Answer from the drawing. Dimensions are ordinates in mm from the lowest x, y and z of the part. A direction names the side the tool comes from. Give positions to 0.01 mm unless a question says otherwise; leave off trailing zeros. Write each loop counter-clockwise with the first axis right and the second up, starting at its lowest first coordinate (ties: lowest second). Pieces come first, ordered by that corner, then holes.
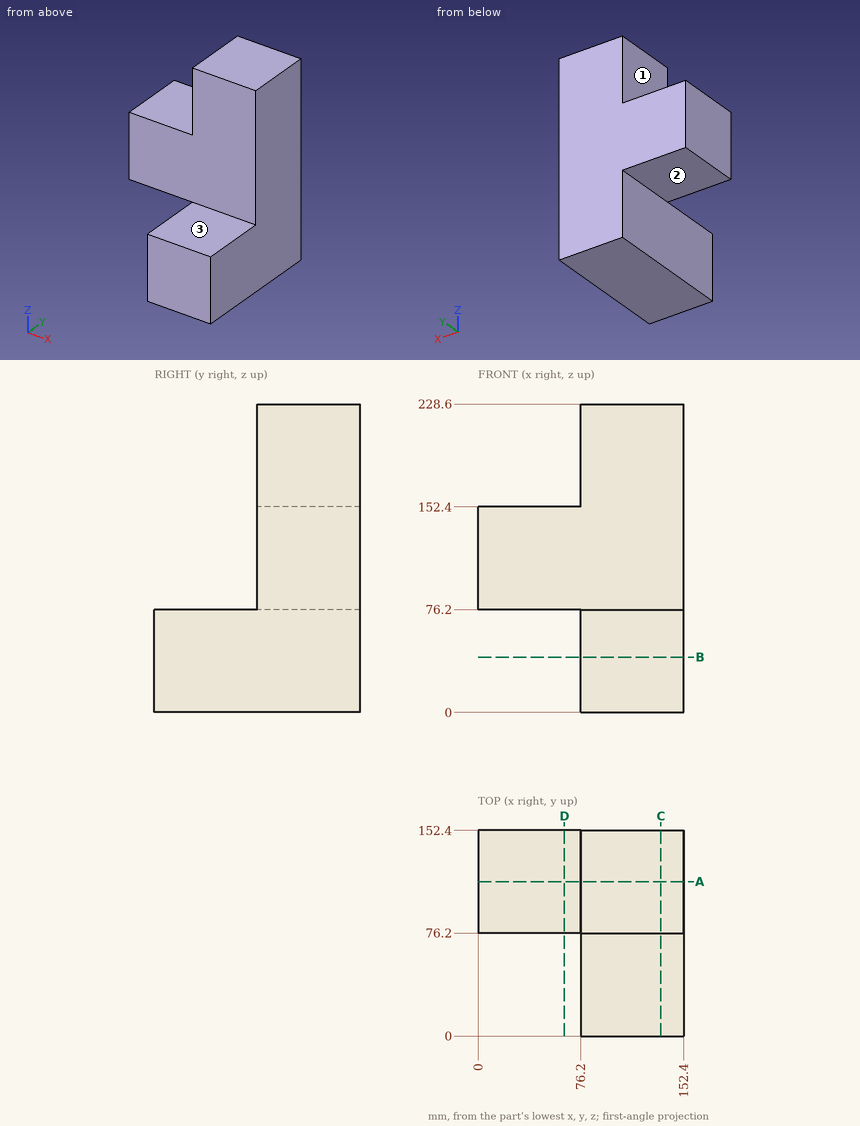
Item 1: Which of the six approach directions +Z, -Z, +X, -X, +Y, -Y give full straight-line access (tool end or side, diameter ignored) to the marked faces 1, 2 and 3?
Result set:
face 1: +Z, -X, +Y, -Y
face 2: -Z, -X, +Y, -Y
face 3: +Z, +X, -X, -Y
Item 2: Section A-A (y = 114.5) is taken. Write down the section's boundary in (x, z).
Result set:
outline: (0, 76.2) - (76.2, 76.2) - (76.2, 0) - (152.4, 0) - (152.4, 228.6) - (76.2, 228.6) - (76.2, 152.4) - (0, 152.4) - close
Item 3: Section D-D (x = 64) is taken. Write down the section's boundary in (y, z), and give its area (3 significant figures).
Result set:
outline: (76.2, 76.2) - (152.4, 76.2) - (152.4, 152.4) - (76.2, 152.4) - close
area: 5,810 mm2
Item 4: Section C-C (x = 135.5) is taken. Write down the section's boundary in (y, z), and give its area (3 significant figures).
Result set:
outline: (0, 0) - (152.4, 0) - (152.4, 228.6) - (76.2, 228.6) - (76.2, 76.2) - (0, 76.2) - close
area: 23,200 mm2
Item 5: Each of these flat-tipped pins is pushed along its axis until it touches: pin 1 Ø8 at (x, z) = (127.5, 174) entering from -Y; pin 2 Ø1.5 at (x, y) = (37, 110.5) entering from +Z; pin 3 Ø23 at (x, y) = (132.5, 31) entering from +Z. Where does it stop, or does it pass through?
Result set:
pin 1: stops at y = 76.2
pin 2: stops at z = 152.4
pin 3: stops at z = 76.2
Item 6: Section B-B (z = 41) is taken. Write down the section's boundary in (x, y).
Result set:
outline: (76.2, 0) - (152.4, 0) - (152.4, 152.4) - (76.2, 152.4) - close
Item 7: Find the intervals of material crossed by line 1 along X through (y, z) = (78, 15.5), in increasing order.
Result set:
line 1: x = 76.2 to 152.4
